CAD build for the part. Positions are in the model's coordinates, mm. A direction names the side the tool comes from. Give positions to 0.01 mm unless a question says otherwise; leave off trailing zeros. Loops run counter-clockwise (first coordinate to the right, second up) from the corner with the lowest first, then second, coordinate; pieces in that order, holes last. Notation, with made-up numbers: M -12.75,31 L 21.25,31 A18 cw 21.25,53 Z; hole C -9,27.25 d10. An arc over 180 degrees is marked long. Answer as CSV lines item,"result".
from build123d import *

# Parameters (mm, degrees)
Y_KSEKLIK_EKSTR_ZYON1_DEPTH = 12


with BuildPart() as part:
    # Çizim1 → Yükseklik-Ekstrüzyon1 (new body)
    with BuildSketch(Plane(origin=(0, 0, 0), x_dir=(1, 0, 0), z_dir=(0, 1, 0))):
        with BuildLine():
            Line((20, 0), (18.5, 0))
            ThreePointArc((18.5, 0), (15.790737726, -6.540737726), (9.25, -9.25))
            ThreePointArc((9.25, -9.25), (15.790737726, -25.040737726), (0, -18.5))
            ThreePointArc((0, -18.5), (-15.790737726, -25.040737726), (-9.25, -9.25))
            ThreePointArc((-9.25, -9.25), (-15.790737726, -6.540737726), (-18.5, 0))
            Line((-18.5, 0), (-20, 0))
            Line((-20, 0), (-20, -22))
            Line((-20, -22), (-24.596747752, -22))
            ThreePointArc((-24.596747752, -22), (0, -33), (24.596747752, -22))
            Line((24.596747752, -22), (20, -22))
            Line((20, -22), (20, 0))
        make_face()
        with BuildLine():
            ThreePointArc((9.25, 9.25), (15.790737726, 6.540737726), (18.5, 0))
            Line((18.5, 0), (20, 0))
            Line((20, 0), (20, 22))
            Line((20, 22), (24.596747752, 22))
            ThreePointArc((24.596747752, 22), (14.378877514, 29.702657818), (1.999081515, 32.939393939))
            ThreePointArc((1.999081515, 32.939393939), (0, 31), (-1.999081515, 32.939393939))
            ThreePointArc((-1.999081515, 32.939393939), (-14.378877514, 29.702657818), (-24.596747752, 22))
            Line((-24.596747752, 22), (-20, 22))
            Line((-20, 22), (-20, 0))
            Line((-20, 0), (-18.5, 0))
            ThreePointArc((-18.5, 0), (-15.790737726, 6.540737726), (-9.25, 9.25))
            ThreePointArc((-9.25, 9.25), (-15.790737726, 25.040737726), (0, 18.5))
            ThreePointArc((0, 18.5), (15.790737726, 25.040737726), (9.25, 9.25))
        make_face()
    extrude(amount=Y_KSEKLIK_EKSTR_ZYON1_DEPTH)


solid = part.part
1) Drill centre lines: line 1 (X direction, y = 4.25, z = -22.5); line 2 (Z direction, x = 9, y = 6.25); line 3 (Z direction, x = -12, y = 3). Where is each one in solid material? Low to high. Write a range as from..to.
Answer below:
line 1,"x = -24.14..-17.59, -0.91..0.91, 17.59..24.14"
line 2,"z = -31.75..-27.75, 27.75..31.75"
line 3,"z = -30.74..-27.33, -9.67..-8.83, 8.83..9.67, 27.33..30.74"
2) Which spindle directions (+Z, -Z, +X, -X, +Y, -Y) get a long thin tool onto all of the face, cutting with end or side? Do faces 1 (the face through (-22, 6, -22)), 2 (the face through (0, 6, -31)), 3 (the face through (20, 6, 0)). Say none if no direction does.
Answer below:
face 1,"-X, +Y, -Y"
face 2,"-Z, +Y, -Y"
face 3,"+X, +Y, -Y"
3) Band-saw the part on C-C on z = -6.5. Give the cut face in (x, y).
Answer below:
outline,"M -20,0 L -15.83,0 L -15.83,12 L -20,12 Z; M 15.83,0 L 20,0 L 20,12 L 15.83,12 Z"
4) Band-saw the part on A-A on x = -14. Give the cut face in (y, z).
Answer below:
outline,"M 0,-29.88 L 12,-29.88 L 12,-26.44 L 0,-26.44 Z; M 0,-10.56 L 12,-10.56 L 12,-7.94 L 0,-7.94 Z; M 0,7.94 L 12,7.94 L 12,10.56 L 0,10.56 Z; M 0,26.44 L 12,26.44 L 12,29.88 L 0,29.88 Z"
5) Mould opens along Z. For faces 4 (the face through (22, 6, 22)), 5 (the face through (-14.22, 5.92, -29.78)), 6 (the face through (14, 12, 10)), 7 (the face through (15.571, 5.916, -25.253)) say: +Z half, -Z half, draft (parallel to the pull), parting line (faces both ways), or undercut.
Answer below:
face 4,"undercut"
face 5,"-Z half"
face 6,"draft"
face 7,"undercut"
6) Band-saw the part on D-D on x = 7. Give the cut face in (y, z).
Answer below:
outline,"M 0,-32.25 L 12,-32.25 L 12,-27.47 L 0,-27.47 Z; M 0,27.47 L 12,27.47 L 12,32.25 L 0,32.25 Z"
7) Flat gauge pins, fed straight in: pin 1 (1.4 mm diameter, centred on x = -22, y = 7.5, fed in from +Z); pin 2 (3.5 mm diameter, centred on x = 23, y = 6, fed in from -Z); pin 3 (2 mm diameter, centred on y = 9, z = -24, fed in from -X); pin 4 (21.5 mm diameter, centred on x = 9.25, z = -18.5, fed in from +Y). Where does each tip first touch, or does it go through?
Answer below:
pin 1,"stops at z = 25.21"
pin 2,"stops at z = -25.25"
pin 3,"stops at x = -23.66"
pin 4,"stops at y = 12"
8) Band-saw the part on B-B on y = 2. Give the cut face in (x, z).
Answer below:
outline,"M -24.6,-22 A33 ccw -2,-32.94 A2 cw 2,-32.94 A33 ccw 24.6,-22 L 20,-22 L 20,22 L 24.6,22 A33 ccw -24.6,22 L -20,22 L -20,-22 Z; hole M -9.25,-9.25 A9.25 ccw long 0,-18.5 A9.25 ccw long 9.25,-9.25 A9.25 ccw 9.25,9.25 A9.25 ccw long 0,18.5 A9.25 ccw long -9.25,9.25 A9.25 ccw Z"
